Part model, mm, in its own coordinate system. A direction names the side the tool comes from. Coordinates: 2 decimals unless noted, no trailing zeros. Write each loop counter-clockwise with the first axis right and the second up, starting at its lowest first coordinate (ties: lowest second). Pieces come first, ordered by that corner, then holes. Notation, with made-up numbers: (64, 76) -> (94, 76) arc R34 ccw to (94, 110) -> close; hole circle Ø1 at (28, -31.5). An arc over 180 degrees is marked (long way). One line per question, with ' | ' between items. Start each with the question number.
Item 1: Saw through at D-D (z = 152.4). List the corners of the cut face in (x, y), and give its area (3 significant figures).
Item 2: Saw through at B-B (x = 15). List the corners of the cut face in (y, z).
Item 3: Probe probe 1 along Z at (x, y) = (1.8, 15); probe 2 along Z at (x, y) = (15, 1.15); probe 3 along Y at (x, z) = (25, 255.5). List the from-to ranges inside material, lowest first. Write a range as [from, to].
Item 4: Saw through at A-A (z = 12.5). List the corners of the cut face in (x, y), and give its area (3 significant figures).
Item 5: Pin check, flat tips, straight feed: pin 1 (9 mm diameter, centred on x = 15, z = 12.5, fed in from +Y); pin 2 (1.5 mm diameter, centred on x = 13.5, z = 127, fed in from -Y); pin 3 (7 mm diameter, centred on y = 15, z = 12.5, fed in from +X); pin 4 (14 mm diameter, centred on y = 23, z = 156.5, fed in from +X). Stop position of each tip, or through.
Item 6: Saw through at C-C (y = 15). List the corners of the cut face in (x, z).
Item 7: 3-axis set-ups, long thin cutter, end or side, ignore diameter. For faces 1 (the cylindrical face through (1.27, 12.05, 15.2)), 2 (the flat face through (2.5, 19, 150)): which of +Z, -Z, +X, -X, +Y, -Y reach the whole face in a straight line?
Item 8: Two-plate mould, pull along Z, no slides. Class faces 3 (the cylindrical face through (16.846, 1.268, 295.849)), 4 (the flat face through (8, 2, 304.8)), 5 (the flat face through (16, 2.5, 150)): pulls with the +Z half, pulls with the -Z half, needs draft (parallel to the pull), parting line crosses it, or undercut.
from build123d import *

# Parameters (mm, degrees)
BOSS_EXTRUDE1_DEPTH = 304.8
SKETCH2_R           = 4
CUT_EXTRUDE1_DEPTH  = 308.50494305
SKETCH3_R           = 4
CUT_EXTRUDE2_DEPTH  = 308.50494305
SKETCH5_R           = 4
CUT_EXTRUDE3_DEPTH  = 308.50494305


with BuildPart() as part:
    # Sketch1 → Boss-Extrude1 (new body)
    with BuildSketch(Plane.XY):
        Polygon((0, 0), (0, 30), (2.5, 30), (2.5, 2.5), (30, 2.5), (30, 0), align=None)
    extrude(amount=BOSS_EXTRUDE1_DEPTH)

    # Sketch2 → Cut-Extrude1 (cut, through all)
    with BuildSketch(Plane(origin=(0, 2.5, 0), x_dir=(1, 0, 0), z_dir=(0, 1, 0))):
        with Locations(Location((15, -12.5, 0), (0, 0, 180))):
            Circle(SKETCH2_R)
        with Locations((15, -292.3)):
            Circle(SKETCH2_R)
    extrude(amount=-CUT_EXTRUDE1_DEPTH, mode=Mode.SUBTRACT)

    # Sketch3 → Cut-Extrude2 (cut, through all)
    with BuildSketch(Plane(origin=(2.5, 0, 0), x_dir=(0, 0, -1), z_dir=(1, 0, 0))):
        with Locations(Location((-12.5, 15, 0), (0, 0, 90))):
            Circle(SKETCH3_R)
        with Locations(Location((-292.3, 15, 0), (0, 0, 270))):
            Circle(SKETCH3_R)
    extrude(amount=-CUT_EXTRUDE2_DEPTH, mode=Mode.SUBTRACT)

    # Sketch5 → Cut-Extrude3 (cut, through all)
    with BuildSketch(Plane(origin=(2.5, 0, 0), x_dir=(0, 0, -1), z_dir=(1, 0, 0))):
        with Locations(Location((-152.4, 15, 0), (0, 0, 90))):
            Circle(SKETCH5_R)
    extrude(amount=-CUT_EXTRUDE3_DEPTH, mode=Mode.SUBTRACT)


solid = part.part
From the geometry:
1) outline: (0, 0) -> (30, 0) -> (30, 2.5) -> (2.5, 2.5) -> (2.5, 11) -> (0, 11) -> close; (0, 19) -> (2.5, 19) -> (2.5, 30) -> (0, 30) -> close | area: 124 mm2
2) outline: (0, 0) -> (2.5, 0) -> (2.5, 8.5) -> (0, 8.5) -> close; (0, 16.5) -> (2.5, 16.5) -> (2.5, 288.3) -> (0, 288.3) -> close; (0, 296.3) -> (2.5, 296.3) -> (2.5, 304.8) -> (0, 304.8) -> close
3) probe 1: [0, 8.5], [16.5, 148.4], [156.4, 288.3], [296.3, 304.8] | probe 2: [0, 8.5], [16.5, 288.3], [296.3, 304.8] | probe 3: [0, 2.5]
4) outline: (0, 0) -> (11, 0) -> (11, 2.5) -> (2.5, 2.5) -> (2.5, 11) -> (0, 11) -> close; (0, 19) -> (2.5, 19) -> (2.5, 30) -> (0, 30) -> close; (19, 0) -> (30, 0) -> (30, 2.5) -> (19, 2.5) -> close | area: 104 mm2
5) pin 1: y = 2.5 | pin 2: y = 0 | pin 3: through | pin 4: x = 2.5
6) outline: (0, 0) -> (2.5, 0) -> (2.5, 8.5) -> (0, 8.5) -> close; (0, 16.5) -> (2.5, 16.5) -> (2.5, 148.4) -> (0, 148.4) -> close; (0, 156.4) -> (2.5, 156.4) -> (2.5, 288.3) -> (0, 288.3) -> close; (0, 296.3) -> (2.5, 296.3) -> (2.5, 304.8) -> (0, 304.8) -> close
7) face 1: +X, -X | face 2: +Z, -Z, +X, +Y
8) face 3: undercut | face 4: pulls with the +Z half | face 5: needs draft
